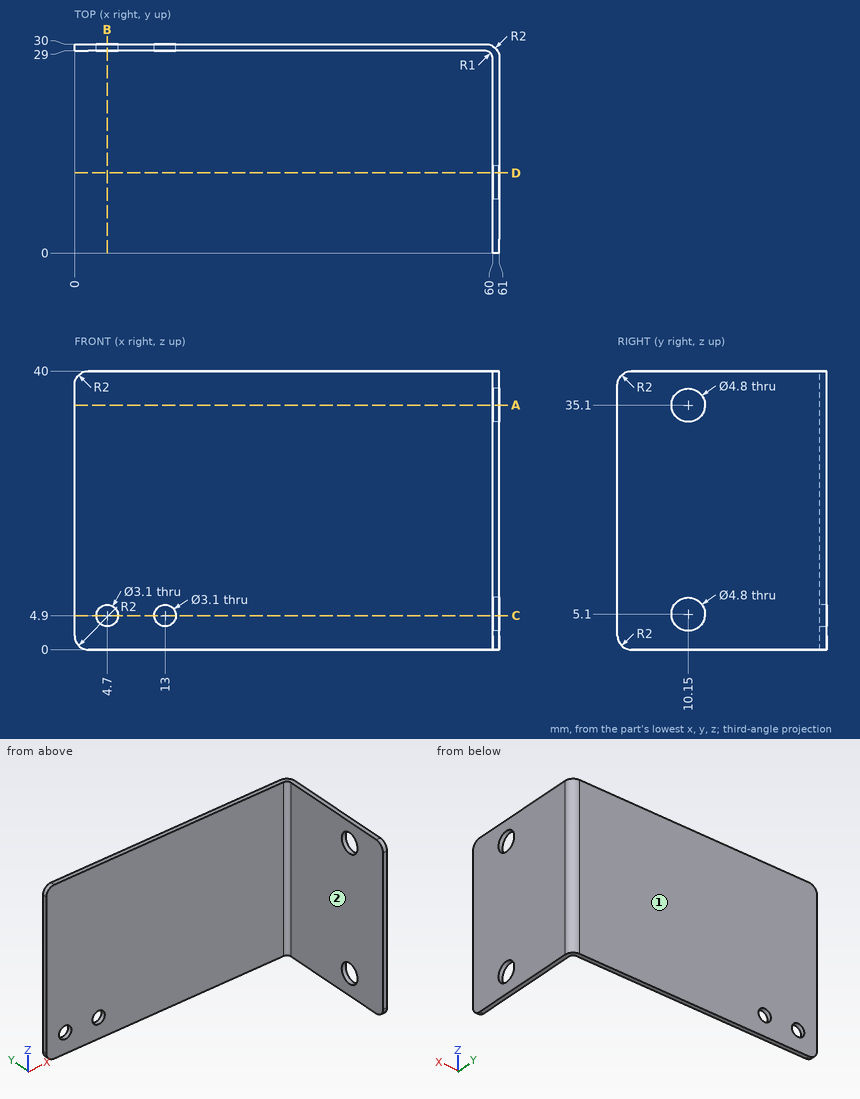
Geometry check sheet. Reference: drawing and pictorial views, mm from the part's lowest x, y, z. A direction names the side the tool comes from. Give positions to 0.01 mm unless a question says otherwise; leave off trailing zeros. Write each loop counter-clockwise with the first axis right and the second up, starting at its lowest first coordinate (ties: lowest second). Pieces come first, ordered by that corner, then holes.
Item 1: Cross-section at B-B (x = 4.7). Enter the section's corners in (y, z).
Item 2: Gauge pin test, flat ends, axial feed: pin 1 (3 mm diameter, centred on x = 4.7, z = 4.9, fed in from -Y); pin 2 (2 mm diameter, centred on x = 38, z = 27.5, fed in from -Y). Record the tip position at first contact, or that the pin passes through.
Item 3: Scan lines: L1, parallel to X at y = 29.5, z = 4.9; L2, parallel to X at y = 2.5, z = 36; L3, parallel to Y at x = 7.5, z = 18.5. Record each from-to range of solid material in increasing order.
Item 4: Cross-section at C-C (z = 4.9). Enter the section's corners in (x, y).
Item 5: Cross-section at D-D (y = 11.5). Enter the section's corners in (x, z).
Item 6: Cross-section at A-A (z = 35.1). Enter the section's corners in (x, y), and give its area (3 significant figures).
Item 7: Access from +Z, -Z, +X, -X, +Y, -Y to the whole of each face (thin tool, end or side, straight path). Record for the marked faces 1 and 2.
Report:
1. outline: (29, 0) - (30, 0) - (30, 3.35) - (29, 3.35) - close; (29, 6.45) - (30, 6.45) - (30, 40) - (29, 40) - close
2. pin 1: passes through
2. pin 2: stops at y = 29
3. L1: x = 0 to 3.15, 6.25 to 11.45, 14.55 to 60.32
3. L2: x = 60 to 61
3. L3: y = 29 to 30
4. outline: (0, 29) - (3.15, 29) - (3.15, 30) - (0, 30) - close; (6.25, 29) - (11.45, 29) - (11.45, 30) - (6.25, 30) - close; (14.55, 29) - (59, 29) arc R1 cw to (60, 28) - (60, 12.54) - (61, 12.54) - (61, 28) arc R2 ccw to (59, 30) - (14.55, 30) - close; (60, 0) - (61, 0) - (61, 7.76) - (60, 7.76) - close
5. outline: (60, 0) - (61, 0) - (61, 3.12) - (60, 3.12) - close; (60, 7.08) - (61, 7.08) - (61, 33.12) - (60, 33.12) - close; (60, 37.08) - (61, 37.08) - (61, 40) - (60, 40) - close
6. outline: (0, 29) - (59, 29) arc R1 cw to (60, 28) - (60, 12.55) - (61, 12.55) - (61, 28) arc R2 ccw to (59, 30) - (0, 30) - close; (60, 0) - (61, 0) - (61, 7.75) - (60, 7.75) - close
6. area: 84.6 mm2
7. face 1: +Z, -Z, +X, -X, +Y
7. face 2: +Z, -Z, -X, -Y
